from build123d import *

# Parameters (mm, degrees)
SKETCH_1_R          = 16.1
EXTRUDE_1_DEPTH     = 2.5
CUT_EXTRUDE_1_DEPTH = 23.905676152
SKETCH_3_W          = 7.1
SKETCH_3_H          = 0.4
CUT_EXTRUDE_2_DEPTH = 23.905676152
CHAMFER_1_SIZE      = 1
CHAMFER_1_SIZE2     = 0.363970234
CHAMFER_2_SIZE      = 0.5
CHAMFER_2_SIZE2     = 1.37373871


with BuildPart() as part:
    # Эскиз1 → Бобышка-Вытянуть1 (new body)
    with BuildSketch(Plane(origin=(0, 0, 0), x_dir=(1, 0, 0), z_dir=(0, 1, 0))):
        with Locations(Location((0, 0, 0), (0, 0, 270))):
            Circle(SKETCH_1_R)
    extrude(amount=EXTRUDE_1_DEPTH)

    # Эскиз2 → Вырез-Вытянуть1 (cut, through all)
    with BuildSketch(Plane(origin=(0, 2.5, 0), x_dir=(1, 0, 0), z_dir=(0, 1, 0))):
        Polygon((0, 10.392304845), (-9, 5.196152423), (-9, -5.196152423), (0, -10.392304845), (9, -5.196152423), (9, 5.196152423), align=None)
    extrude(amount=-CUT_EXTRUDE_1_DEPTH, mode=Mode.SUBTRACT)

    # Эскиз3 → Вырез-Вытянуть2 (cut, through all)
    with BuildSketch(Plane(origin=(0, 2.5, 0), x_dir=(1, 0, 0), z_dir=(0, 1, 0))):
        with Locations((-12.55, 0)):
            Rectangle(SKETCH_3_W, SKETCH_3_H)
    extrude(amount=-CUT_EXTRUDE_2_DEPTH, mode=Mode.SUBTRACT)

    # Фаска1
    chamfer_1_edges = [part.edges().sort_by_distance(p)[0] for p in [
        (11.45491161, 0, -11.313487526),
    ]]
    chamfer_1_side = [part.faces().sort_by_distance(p)[0] for p in [
        (11.45491161, 1.25, -11.313487526),
    ]]
    chamfer(chamfer_1_edges, length=CHAMFER_1_SIZE, length2=CHAMFER_1_SIZE2, reference=chamfer_1_side[0])

    # Фаска2
    chamfer_2_edges = [part.edges().sort_by_distance(p)[0] for p in [
        (4.5, 0, -7.794228634),
        (9, 0, 0),
        (4.5, 0, 7.794228634),
        (-4.5, 0, 7.794228634),
        (-9, 0, -2.698076211),
        (-4.5, 0, -7.794228634),
        (-9, 0, 2.698076211),
    ]]
    chamfer_2_side = [part.faces().sort_by_distance(p)[0] for p in [
        (-12.367379373, 0, -0.245073147),
    ]]
    chamfer(chamfer_2_edges, length=CHAMFER_2_SIZE, length2=CHAMFER_2_SIZE2, reference=chamfer_2_side[0])


solid = part.part
Work out the finished part from the listing and answer in its coordinate system (mm). A direction names the side the tool comes from. Round coordinates to 2 decimals unless told otherwise and drop trailing zeros. Order: outer loops, then holes, each group sorted by start corner. A loop starts at its lowest first (then second) coordinate and runs counter-clockwise, first axis right, second up. Notation, with made-up numbers: M 74,57.25 L 84,57.25 A11 ccw 84,70.25 Z; hole C 49.5,-28.5 d8. An arc over 180 degrees is marked long. Put each result on its own line as item: value. Start each with the question number.
Q1. Section A-A, the plane y = 2.1 is taken. Write down the section's boundary in (x, z), and give its area (3 significant figures).
Q2. A tool of negligible diameter and unlimited length cuts with its end or side. For faces 1 (the flat face through (-4.557, 0.696, -8.046)), 2 (the flat face through (-4.56, 1.94, 7.76)), 3 (the flat face through (-13, 1, 0.2)), from which of +Z, -Z, +X, -X, +Y, -Y can it reach the whole face along a straight path? Write none if from no direction.
Q3. Straight lines are drawn through the part: L1, parallel to Z at x = 5, y = 2.3; L2, parallel to X at y = 1.45, z = 2; L3, parallel to Z at x = -8, y = 2.35. For each, find the intervals that lie inside material, in ascending order. Write a range as [from, to].
Q4. Section B-B, the plane y = 0.5 is taken. Write down the section's boundary in (x, z), and give its area (3 significant figures).
Q5. Flat-ended cylindrical pins translate along their axes: pin 1 (0.9 mm diameter, centred on y = 2, z = 2, fed in from -X); pin 2 (1.3 mm diameter, centred on x = -12, y = 1, fed in from +Z); pin 3 (0.6 mm diameter, centred on y = 2, z = 2, fed in from +X). Find the tip coordinate at first contact, or state that the pin passes through.
Q6. For a pull along Z with two mould halves and no side action, classify faces 4 (the conical face through (15.78, 0.16, 0.69)), 5 (the flat face through (-9, 2, 3)), 6 (the flat face through (-7, 2.5, 7)) as pulls with the +Z half, pulls with the -Z half, needs draft (parallel to the pull), parting line crosses it, or undercut.
Findings below:
1. outline: M -16.1,-0.2 A16.1 ccw long -16.1,0.2 L -9,0.2 L -9,5.2 L 0,10.39 L 9,5.2 L 9,-5.2 L 0,-10.39 L -9,-5.2 L -9,-0.2 Z
1. area: 531 mm^2
2. face 1: -Y
2. face 2: +Y, -Y
2. face 3: -X, +Y, -Y
3. L1: z = [-15.3, -7.51], [7.51, 15.3]
3. L2: x = [-15.98, -9], [9, 15.98]
3. L3: z = [-13.97, -5.77], [5.77, 13.97]
4. outline: M -15.92,-0.2 A15.92 ccw long -15.92,0.2 L -9.32,0.2 L -9.32,5.38 L 0,10.76 L 9.32,5.38 L 9.32,-5.38 L 0,-10.76 L -9.32,-5.38 L -9.32,-0.2 Z
4. area: 493 mm^2
5. pin 1: stops at x = -16.03
5. pin 2: stops at z = 11.42
5. pin 3: stops at x = 16.01
6. face 4: parting line crosses it
6. face 5: undercut
6. face 6: needs draft
